```python
from build123d import *

# Parameters (mm, degrees)
BOSS_EXTRUDE1_DEPTH     = 9
SKETCH2_R               = 1.75
CUT_EXTRUDE1_DEPTH      = 11.651759691
CUT_EXTRUDE1_DEPTH_BACK = 10.276217487
SKETCH3_R               = 3.5
CUT_EXTRUDE2_DEPTH      = 5.5
SKETCH4_R               = 3.5
CUT_EXTRUDE3_DEPTH      = 7
SKETCH5_R               = 1.5
CUT_EXTRUDE4_DEPTH      = 10.0000001


with BuildPart() as part:
    # Sketch1 → Boss-Extrude1 (new body)
    with BuildSketch(Plane(origin=(0, 0, 0), x_dir=(1, 0, 0), z_dir=(0, 1, 0))):
        with BuildLine():
            ThreePointArc((9, 0), (0.040582687, 8.999908502), (-8.99963401, 0.081164549))
            Line((-8.99963401, 0.081164549), (-4.25, 0))
            ThreePointArc((-4.25, 0), (0, 4.25), (4.25, 0))
            ThreePointArc((4.25, 0), (0.585435043, -4.209485219), (-4.088713322, -1.159708311))
            Line((-4.088713322, -1.159708311), (-8.837484751, -1.702604851))
            ThreePointArc((-8.837484751, -1.702604851), (0.855171691, -8.959279066), (9, 0))
        make_face()
    extrude(amount=BOSS_EXTRUDE1_DEPTH)

    # Sketch2 → Cut-Extrude1 (cut, two sides)
    with BuildSketch(Plane(origin=(0.078121964, 0, 0.683340793), x_dir=(-0.993528428, 0, 0.113583725), z_dir=(-0.113583725, 0, -0.993528428))) as cut_extrude1_sk:
        with Locations((6.583828722, 4.5)):
            Circle(SKETCH2_R)
    extrude(amount=CUT_EXTRUDE1_DEPTH, mode=Mode.SUBTRACT)
    extrude(cut_extrude1_sk.sketch, amount=-CUT_EXTRUDE1_DEPTH_BACK, mode=Mode.SUBTRACT)

    # Sketch3 → Cut-Extrude2 (cut)
    with BuildSketch(Plane.XY.offset(10)):
        with Locations((-5.798386902, 4.384929451)):
            Circle(SKETCH3_R)
    extrude(amount=-CUT_EXTRUDE2_DEPTH, mode=Mode.SUBTRACT)

    # Sketch4 → Cut-Extrude3 (cut)
    with BuildSketch(Plane.XY.offset(-10)):
        with Locations((-7.26360584, 4.480644852)):
            Circle(SKETCH4_R)
    extrude(amount=CUT_EXTRUDE3_DEPTH, mode=Mode.SUBTRACT)

    # Sketch5 → Cut-Extrude4 (cut, through all)
    with BuildSketch(Plane(origin=(0, 9, 0), x_dir=(1, 0, 0), z_dir=(0, 1, 0))):
        with Locations((0.035505664, -6.484233459)):
            Circle(SKETCH5_R)
        with Locations((0, 6.625)):
            Circle(SKETCH5_R)
    extrude(amount=-CUT_EXTRUDE4_DEPTH, mode=Mode.SUBTRACT)


solid = part.part
```
Can you work these out from the model? Positions are in its coordinate system, mm. A direction names the side the tool comes from. Round coordinates to 2 decimals unless told otherwise and drop trailing zeros. Order: outer loops, then holes, each group sorted by start corner. A loop starts at its lowest first (then second) coordinate and runs counter-clockwise, first axis right, second up. Notation, with made-up numbers: (-4, -15) -> (52, -15) arc R16 ccw to (52, -6) -> close; hole circle Ø4 at (49.25, -7). An arc over 180 degrees is marked (long way). Return JSON: item names as keys, results as strings. Group by question number.
1. If we section it at B-B, the plane x = -0.75: Write out the boundary of the cut face in (y, z), then the cut area to 3 significant figures.
2. If we section it at A-A, the plane y = 6: Count the separate pieces of the cut face and the enclosed holes in it, then the cut area to 3 significant figures.
3. Which directions (+Z, -Z, +X, -X, +Y, -Y) give clear straight access to the entire face, cutting with the end or side of a thin tool? Please do faces 4 (the face through (-4.54, 4.58, 2.85)), 5 (the face through (-4, 4, 4.5)).
4. Will these pins go through, and if not, where does the flat tip stop? pin 1 (1.5 mm diameter, centred on x = 4, y = 5.5, fed in from +Z); pin 2 (1 mm diameter, centred on x = 3.5, y = 3.5, fed in from +Z); pin 3 (1.5 mm diameter, centred on x = -4, y = 2, fed in from -Z).
5. I need wall thicknesses on line 1 (Z direction, x = 0, y = 6.25) (3 decimals); line 2 (X direction, y = 6, z = -2); line 3 (Z direction, x = 1.25, y = 1). Which ranges of each line are inside material? Lowest first, please. Write a range as [from, to].
6. If we section it at C-C, the plane z = -7.25: Write out the boundary of the cut face in (x, y).
7. We'd pull the mould along X, two halves only. Please class faces 1 (the face through (-2.3, 4.3, 6.2)), 2 (the face through (-4.847, 3.437, 1.246)), 3 (the face through (4, 0, 2)): released by +X, released by -X, zero draft, split by the parting line, or undercut.
Output values:
{
 "1": {"outline": "(0, -8.97) -> (9, -8.97) -> (9, -7.92) -> (0, -7.92) -> close; (0, -5.33) -> (9, -5.33) -> (9, -4.18) -> (0, -4.18) -> close; (0, 4.18) -> (9, 4.18) -> (9, 5.21) -> (0, 5.21) -> close; (0, 7.76) -> (9, 7.76) -> (9, 8.97) -> (0, 8.97) -> close", "area": "39.8 mm²"},
 "2": {"separate pieces": "3", "enclosed holes": "2", "area": "139 mm²"},
 "3": {"face 4": "none", "face 5": "+Z"},
 "4": {"pin 1": "z = 8.39", "pin 2": "z = 8.49", "pin 3": "z = -8.39"},
 "5": {"line 1": "[-9, -8.125], [-5.125, -4.25], [4.25, 4.985], [7.984, 9]", "line 2": "[-8.77, -7.76], [-5.95, -3.75], [3.75, 8.77]", "line 3": "[-8.91, -7.45], [-5.8, -4.06], [4.06, 5.6], [7.36, 8.91]"},
 "6": {"outline": "(-5.33, 0) -> (-1.36, 0) -> (-1.36, 9) -> (-5.33, 9) -> (-5.33, 7.4) arc R3.5 cw to (-5.33, 1.56) -> close; (1.36, 0) -> (5.33, 0) -> (5.33, 9) -> (1.36, 9) -> close"},
 "7": {"face 1": "undercut", "face 2": "released by -X", "face 3": "zero draft"}
}
